Source: CAD feature listing. Evaluate the final solid. Frame: model axes, mm. Face numbers are marked on the shaded views. A direction names the side the tool comes from. Give positions to 0.01 mm unless a question says otherwise; leave off trailing zeros. Order: outer loops, then holes, each group sorted by start corner. A loop starts at its lowest first (then second) coordinate and runs counter-clockwise, first axis right, second up. Notation, with made-up numbers: M 80,-20.5 L 133,-20.5 A32 cw 133,14.5 Z; hole C 23,11.25 d6. An arc over 180 degrees is marked long. Return JSON: item names as keys, results as strings.
from build123d import *

# Parameters (mm, degrees)
CYLINDER001_R     = 3
CYLINDER001_DEPTH = 148
BOX007_W          = 16
BOX007_H          = 6
BOX007_DEPTH      = 10
CYLINDER_R        = 3
CYLINDER_DEPTH    = 148
BOX006_W          = 16
BOX006_H          = 6
BOX006_DEPTH      = 10
BOX005_W          = 12
BOX005_H          = 10
BOX005_DEPTH      = 20
BOX003_W          = 25
BOX003_H          = 25
BOX003_DEPTH      = 15
BOX001_W          = 145
BOX001_H          = 170
BOX001_DEPTH      = 200
BOX_W             = 155
BOX_H             = 180
BOX_DEPTH         = 170
BOX004_W          = 4
BOX004_H          = 50
BOX004_DEPTH      = 25
BOX002_W          = 155
BOX002_H          = 180
BOX002_DEPTH      = 10


with BuildPart() as cylinder001:
    # Cylinder001 → Cylinder001 (new body)
    with BuildSketch(Plane(origin=(7, 139, 175), x_dir=(1, 0, 0), z_dir=(0, -1, 0))):
        Circle(CYLINDER001_R)
    extrude(amount=CYLINDER001_DEPTH)


with BuildPart() as obj1:
    # Box007 → Box007 (new body)
    with BuildSketch(Plane.XY.offset(170)):
        with Locations((8, 3)):
            Rectangle(BOX007_W, BOX007_H)
    extrude(amount=BOX007_DEPTH)

    # Cut004: cut Cylinder001
    add(cylinder001.part, mode=Mode.SUBTRACT)


with BuildPart() as cylinder:
    # Cylinder → Cylinder (new body)
    with BuildSketch(Plane(origin=(7, 192, 175), x_dir=(1, 0, 0), z_dir=(0, -1, 0))):
        Circle(CYLINDER_R)
    extrude(amount=CYLINDER_DEPTH)


with BuildPart() as obj2:
    # Box006 → Box006 (new body)
    with BuildSketch(Plane(origin=(0, 174, 170), x_dir=(1, 0, 0), z_dir=(0, 0, 1))):
        with Locations((8, 3)):
            Rectangle(BOX006_W, BOX006_H)
    extrude(amount=BOX006_DEPTH)

    # Cut003: cut Cylinder
    add(cylinder.part, mode=Mode.SUBTRACT)


with BuildPart() as cube003:
    # Box005 → Box005 (new body)
    with BuildSketch(Plane(origin=(146, 85, 130), x_dir=(1, 0, 0), z_dir=(0, 0, 1))):
        with Locations((6, 5)):
            Rectangle(BOX005_W, BOX005_H)
    extrude(amount=BOX005_DEPTH)


with BuildPart() as agujero:
    # Box003 → Box003 (new body)
    with BuildSketch(Plane(origin=(10, -7, 5), x_dir=(1, 0, 0), z_dir=(0, 0, 1))):
        with Locations((12.5, 12.5)):
            Rectangle(BOX003_W, BOX003_H)
    extrude(amount=BOX003_DEPTH)


with BuildPart() as cube001:
    # Box001 → Box001 (new body)
    with BuildSketch(Plane(origin=(5, 5, 5), x_dir=(1, 0, 0), z_dir=(0, 0, 1))):
        with Locations((72.5, 85)):
            Rectangle(BOX001_W, BOX001_H)
    extrude(amount=BOX001_DEPTH)


with BuildPart() as fusion002:
    # Box → Box (new body)
    with BuildSketch(Plane.XY):
        with Locations((77.5, 90)):
            Rectangle(BOX_W, BOX_H)
    extrude(amount=BOX_DEPTH)

    # Cut: cut Cube001
    add(cube001.part, mode=Mode.SUBTRACT)

    # Cut001: cut Agujero
    add(agujero.part, mode=Mode.SUBTRACT)

    # Cut002: cut Cube003
    add(cube003.part, mode=Mode.SUBTRACT)

    # Fusion001: union obj2
    add(obj2.part)

    # Fusion002: union obj1
    add(obj1.part)


with BuildPart() as cube002:
    # Box004 → Box004 (new body)
    with BuildSketch(Plane(origin=(155, 65, 155), x_dir=(1, 0, 0), z_dir=(0, 0, 1))):
        with Locations((2, 25)):
            Rectangle(BOX004_W, BOX004_H)
    extrude(amount=BOX004_DEPTH)


with BuildPart() as tapa:
    # Box002 → Box002 (new body)
    with BuildSketch(Plane.XY.offset(170)):
        with Locations((77.5, 90)):
            Rectangle(BOX002_W, BOX002_H)
    extrude(amount=BOX002_DEPTH)

    # Fusion: union Cube002
    add(cube002.part)

    # Cut005: cut Fusion002
    add(fusion002.part, mode=Mode.SUBTRACT)


solid = tapa.part
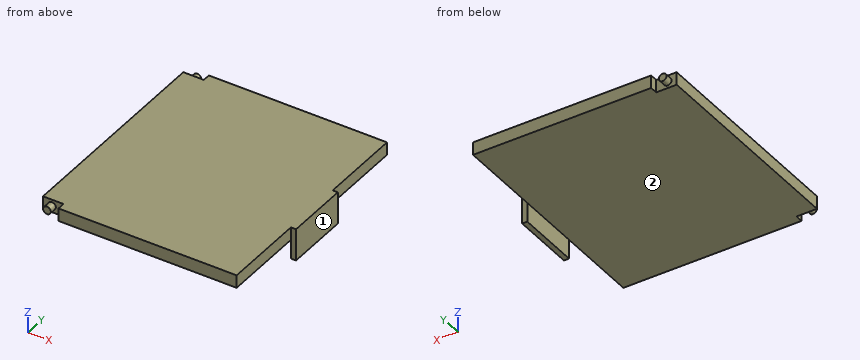
1. Ray query, probe 1 along Z at (x, y) = (115.5, 40); probe 2 along X at (y, z) = (31, 171); probe 3 along X at (y, z) = (110, 161.25). Return the intervals inside material, ascending.
Evaluation:
{"probe 1": "z = 170 to 180", "probe 2": "x = 0 to 155", "probe 3": "x = 155 to 159"}
2. First-contact query: pin 1 (1.5 mm diameter, centred on x = 55.5, y = 97.5, fed in from -Z); pin 2 (7.5 mm diameter, centred on y = 83.5, z = 162.5, fed in from -X); pin 3 (1 mm diameter, centred on y = 49.5, z = 175.5, fed in from +X). Flat tips, straight axial feed; report the tip coordinate or a pass-through.
Evaluation:
{"pin 1": "stops at z = 170", "pin 2": "stops at x = 155", "pin 3": "stops at x = 155"}
3. Set-up query: the marked faces 1 and 2. Return all of +Z, -Z, +X, -X, +Y, -Y with unobstructed straight access to the full face (end or side cutting, diameter ignored); none if empty.
Evaluation:
{"face 1": "+Z, -Z, +X, +Y, -Y", "face 2": "-Z, -X, +Y, -Y"}
4. Section query D-D (z = 165). Return loops of the section in (x, y).
Evaluation:
{"outline": "M 155,65 L 159,65 L 159,115 L 155,115 Z"}
5. Section query B-B (x = 7). Return loops of the section in (y, z).
Evaluation:
{"outline": "M 0,172 L 6,172 L 6,170 L 174,170 L 174,172 L 180,172 L 180,178 L 174,178 L 174,180 L 6,180 L 6,178 L 0,178 Z"}
6. Section query A-A (z = 175). Return loops of the section in (x, y), then the cut area to 3 significant figures.
Evaluation:
{"outline": "M 0,6 L 4,6 L 4,0 L 10,0 L 10,6 L 16,6 L 16,0 L 155,0 L 155,65 L 159,65 L 159,115 L 155,115 L 155,180 L 16,180 L 16,174 L 10,174 L 10,180 L 4,180 L 4,174 L 0,174 Z", "area": "28,000 mm^2"}
7. Section query C-C (y = 83). Return loops of the section in (x, z).
Evaluation:
{"outline": "M 0,170 L 155,170 L 155,155 L 159,155 L 159,180 L 0,180 Z"}
